```python
from build123d import *

# Parameters (mm, degrees)
SKETCH1_R            = 53.5
BOSS_EXTRUDE1_DEPTH  = 2
SKETCH2_R            = 53.5
SKETCH2_R_2          = 51.6
BOSS_EXTRUDE2_DEPTH  = 10
BOSS_EXTRUDE3_START  = 9
SKETCH4_R            = 53.5
BOSS_EXTRUDE3_DEPTH  = 9
SKETCH6_W            = 36
SKETCH6_H            = 36
CUT_EXTRUDE1_DEPTH   = 6.5
CUT_EXTRUDE2_START   = -36
CUT_EXTRUDE2_DEPTH   = 36
CUT_EXTRUDE2_2_DEPTH = 36
CUT_EXTRUDE2_START_2 = -19
CUT_EXTRUDE2_3_DEPTH = 38
SKETCH14_R           = 2.35
CUT_EXTRUDE3_DEPTH   = 4
SKETCH15_W           = 36
SKETCH15_H           = 71.5
CUT_EXTRUDE4_DEPTH   = 2


with BuildPart() as part:
    # Sketch1 → Boss-Extrude1 (new body)
    with BuildSketch(Plane(origin=(0, 0, 0), x_dir=(1, 0, 0), z_dir=(0, 1, 0))):
        with Locations(Location((0, 0, 0), (0, 0, 270))):
            Circle(SKETCH1_R)
    extrude(amount=BOSS_EXTRUDE1_DEPTH)

    # Sketch2 → Boss-Extrude2 (add)
    with BuildSketch(Plane(origin=(0, 2, 0), x_dir=(1, 0, 0), z_dir=(0, 1, 0))):
        with Locations(Location((0, 0, 0), (0, 0, 270))):
            Circle(SKETCH2_R)
        with Locations(Location((0, 0, 0), (0, 0, 270))):
            Circle(SKETCH2_R_2, mode=Mode.SUBTRACT)
    extrude(amount=BOSS_EXTRUDE2_DEPTH)

    # Sketch4 → Boss-Extrude3 (add)
    with BuildSketch(Plane.XZ.offset(BOSS_EXTRUDE3_START)):
        with Locations(Location((0, 0, 0), (0, 0, 270))):
            Circle(SKETCH4_R)
    extrude(amount=-BOSS_EXTRUDE3_DEPTH)

    # Sketch6 → Cut-Extrude1 (cut)
    with BuildSketch(Plane.XZ.offset(9)):
        Rectangle(SKETCH6_W, SKETCH6_H)
    extrude(amount=-CUT_EXTRUDE1_DEPTH, mode=Mode.SUBTRACT)

    # Cut-Extrude2: read off the stored shape, not the designer's step
    # Cut-Extrude2 outline → Cut-Extrude2 (cut)
    with BuildSketch(Plane.XY.offset(-18).offset(CUT_EXTRUDE2_START)):
        Polygon((15.634193477, -9), (18, -2.5), (-18, -2.5), (-15.634193477, -9), align=None)
    extrude(amount=CUT_EXTRUDE2_DEPTH, mode=Mode.SUBTRACT)

    # Cut-Extrude2 2 outline → Cut-Extrude2 2 (add)
    with BuildSketch(Plane.XY.offset(-18)):
        Polygon((18, -9), (18, -2.5), (15.634193477, -9), align=None)
        Polygon((-15.634193477, -9), (-18, -2.5), (-18, -9), align=None)
    extrude(amount=CUT_EXTRUDE2_2_DEPTH)

    # Cut-Extrude2 3 outline → Cut-Extrude2 3 (add)
    with BuildSketch(Plane.YZ.offset(CUT_EXTRUDE2_START_2)):
        Polygon((-9, 18), (-9, 15.634193477), (-2.5, 18), align=None)
    extrude(amount=CUT_EXTRUDE2_3_DEPTH)

    # Sketch14 → Cut-Extrude3 (cut)
    with BuildSketch(Plane.XZ.offset(2.5)):
        with Locations(Location((0, -37, 0), (0, 0, 270))):
            Circle(SKETCH14_R)
    extrude(amount=-CUT_EXTRUDE3_DEPTH, mode=Mode.SUBTRACT)

    # Sketch15 → Cut-Extrude4 (cut)
    with BuildSketch(Plane.XZ.offset(2.5)):
        with Locations((0, -17.75)):
            Rectangle(SKETCH15_W, SKETCH15_H)
    extrude(amount=-CUT_EXTRUDE4_DEPTH, mode=Mode.SUBTRACT)


solid = part.part
```
The model under review builds one solid part; all positions refer to its coordinate system, in mm. A direction names the side the tool comes from. Coordinates: 2 decimals unless noted, no trailing zeros. Write each loop counter-clockwise with the first axis right and the second up, starting at its lowest first coordinate (ties: lowest second). Pieces come first, ordered by that corner, then holes.
1) Clearance check with flat-ended pins moving along their axes: pin 1 Ø6 at (y, z) = (0.5, 9) entering from -X; pin 2 Ø5 at (x, z) = (-27, 40) entering from +Y; pin 3 Ø6 at (y, z) = (5.5, -34.5) entering from -X. State where each tip first meets the part, or that it passes through.
2) We need section A-A on x = 0. State the section outline as (y, z) points, then the cut area to 3 significant figures.
3) We need section D-D on z = 21. State the section outline as (x, y) points.
4) To check wall thickness, follow probe 1 along X at (y, z) = (4.75, 0.5); probe 2 along Y at (x, z) = (-1.5, -33); probe 3 along X at (y, z) = (0.2, -37). State the ranges of each line that lie inside material, in increasing order.
5) Machinability: for faces 1 (the face through (0, 1.5, -37)), 2 (the face through (-0.3, -5.8, 16.8)), 3 (the face through (-50.373, 6.93, -11.186)), which of the approach directions +Z, -Z, +X, -X, +Y, -Y give a long, thin tool a straight path to every point of the face, cutting with its end or side? Answer none if there is none.
6) We need section C-C on y = 10.5. State the section outline as (x, z) points.
7) The part is to be moulded in two halves that separate along Z. For faces 4 (the face through (1, 2, -1)), 5 (the face through (53.384, -0.98, -3.527)), 6 (the face through (0, -0.5, -17)), 7 (the face through (0.71, 0.49, -39.24)), say which applies: pulls with the +Z half, pulls with the -Z half, needs draft (parallel to the pull), parting line crosses it, or undercut.
8) We need section B-B on z = 0. State the section outline as (x, y) points, then the cut area to 3 significant figures.
Answer list:
1. pin 1: stops at x = -53.16
1. pin 2: stops at y = 2
1. pin 3: stops at x = -43.24
2. outline: (-9, 15.63) - (-2.5, 18) - (-0.5, 18) - (-0.5, -34.65) - (1.5, -34.65) - (1.5, -39.35) - (-0.5, -39.35) - (-0.5, -53.5) - (12, -53.5) - (12, -51.6) - (2, -51.6) - (2, 51.6) - (12, 51.6) - (12, 53.5) - (-9, 53.5) - close
2. area: 606 mm2
3. outline: (-49.21, -9) - (49.21, -9) - (49.21, 12) - (47.13, 12) - (47.13, 2) - (-47.13, 2) - (-47.13, 12) - (-49.21, 12) - close
4. probe 1: x = -53.5 to -51.6, 51.6 to 53.5
4. probe 2: y = -0.5 to 2
4. probe 3: x = -38.64 to -2.35, 2.35 to 38.64
5. face 1: -Y
5. face 2: -Z
5. face 3: +Y
6. outline: circle Ø107 at (0, 0); hole circle Ø103.2 at (0, 0)
7. face 4: undercut
7. face 5: parting line crosses it
7. face 6: needs draft
7. face 7: undercut
8. outline: (-53.5, -9) - (-15.63, -9) - (-18, -2.5) - (-18, -0.5) - (18, -0.5) - (18, -2.5) - (15.63, -9) - (53.5, -9) - (53.5, 12) - (51.6, 12) - (51.6, 2) - (-51.6, 2) - (-51.6, 12) - (-53.5, 12) - close
8. area: 924 mm2
